```python
from build123d import *

# Parameters (mm, degrees)
SKETCH1_W           = 50
SKETCH1_H           = 39
BOSS_EXTRUDE1_DEPTH = 3
SKETCH2_W           = 2
SKETCH2_H           = 2
SKETCH2_H_2         = 8
SKETCH2_W_2         = 8
SKETCH2_W_3         = 10
SKETCH2_H_3         = 10
BOSS_EXTRUDE2_DEPTH = 5
SKETCH3_W           = 44
SKETCH3_H           = 28
CUT_EXTRUDE1_DEPTH  = 5
SKETCH4_W           = 2
SKETCH4_H           = 2
SKETCH4_H_2         = 5.5
SKETCH4_W_2         = 5.5
BOSS_EXTRUDE3_DEPTH = 5
SKETCH5_W           = 2
SKETCH5_H           = 5.5
SKETCH5_H_2         = 2
SKETCH5_W_2         = 5.5
BOSS_EXTRUDE4_DEPTH = 5
SKETCH6_W           = 38
SKETCH6_H           = 17
CUT_EXTRUDE2_DEPTH  = 5
SKETCH7_W           = 35
SKETCH7_H           = 24
CUT_EXTRUDE3_DEPTH  = 5


with BuildPart() as part:
    # Sketch1 → Boss-Extrude1 (new body)
    with BuildSketch(Plane.XY):
        Polygon((5, 47), (0, 47), (0, 0), (63, 0), (63, 47), (58, 47), align=None)
        Polygon((5, 79), (5, 47), (58, 47), (58, 79), (56.5, 79), (6.5, 79), align=None)
        with Locations((31.5, 98.5)):
            Rectangle(SKETCH1_W, SKETCH1_H)
    extrude(amount=BOSS_EXTRUDE1_DEPTH)

    # Sketch2 → Boss-Extrude2 (add)
    with BuildSketch(Plane.XY.offset(3)):
        Polygon((53, 45), (61, 45), (61, 47), (58, 47), (53, 47), align=None)
        with Locations((62, 46)):
            Rectangle(SKETCH2_W, SKETCH2_H)
        with Locations((62, 41)):
            Rectangle(SKETCH2_W, SKETCH2_H_2)
        with Locations((62, 6)):
            Rectangle(SKETCH2_W, SKETCH2_H_2)
        with Locations((62, 1)):
            Rectangle(SKETCH2_W, SKETCH2_H)
        with Locations((57, 1)):
            Rectangle(SKETCH2_W_2, SKETCH2_H)
        with Locations((5, 1)):
            Rectangle(SKETCH2_W_3, SKETCH2_H)
        with Locations((5, 46)):
            Rectangle(SKETCH2_W_3, SKETCH2_H)
        with Locations((1, 29)):
            Rectangle(SKETCH2_W, SKETCH2_H_3)
    extrude(amount=BOSS_EXTRUDE2_DEPTH)

    # Sketch3 → Cut-Extrude1 (cut)
    with BuildSketch(Plane.XY.offset(3)):
        with Locations((31.5, 23.5)):
            Rectangle(SKETCH3_W, SKETCH3_H)
    extrude(amount=-CUT_EXTRUDE1_DEPTH, mode=Mode.SUBTRACT)

    # Sketch4 → Boss-Extrude3 (add)
    with BuildSketch(Plane.XY.offset(3)):
        with Locations((6, 48)):
            Rectangle(SKETCH4_W, SKETCH4_H)
        with Locations((6, 51.75)):
            Rectangle(SKETCH4_W, SKETCH4_H_2)
        Polygon((7, 49), (7, 47), (10, 47), (12.5, 47), (12.5, 49), align=None)
        with Locations((6, 74.25)):
            Rectangle(SKETCH4_W, SKETCH4_H_2)
        Polygon((5, 79), (5, 77), (7, 77), (7, 79), (6.5, 79), align=None)
        with Locations((9.75, 78)):
            Rectangle(SKETCH4_W_2, SKETCH4_H)
        with Locations((53.25, 78)):
            Rectangle(SKETCH4_W_2, SKETCH4_H)
        Polygon((56, 77), (58, 77), (58, 79), (56.5, 79), (56, 79), align=None)
        with Locations((57, 74.25)):
            Rectangle(SKETCH4_W, SKETCH4_H_2)
        with Locations((57, 51.75)):
            Rectangle(SKETCH4_W, SKETCH4_H_2)
        with Locations((57, 48)):
            Rectangle(SKETCH4_W, SKETCH4_H)
        Polygon((53, 47), (56, 47), (56, 49), (50.5, 49), (50.5, 47), align=None)
    extrude(amount=BOSS_EXTRUDE3_DEPTH)

    # Sketch5 → Boss-Extrude4 (add)
    with BuildSketch(Plane.XY.offset(3)):
        with Locations((7.5, 83.75)):
            Rectangle(SKETCH5_W, SKETCH5_H)
        Polygon((8.5, 81), (8.5, 79), (12.5, 79), (14, 79), (14, 81), align=None)
        with Locations((7.5, 80)):
            Rectangle(SKETCH5_W, SKETCH5_H_2)
        Polygon((54.5, 79), (54.5, 81), (49, 81), (49, 79), (50.5, 79), align=None)
        with Locations((55.5, 80)):
            Rectangle(SKETCH5_W, SKETCH5_H_2)
        with Locations((55.5, 83.75)):
            Rectangle(SKETCH5_W, SKETCH5_H)
        with Locations((51.75, 117)):
            Rectangle(SKETCH5_W_2, SKETCH5_H_2)
        with Locations((55.5, 117)):
            Rectangle(SKETCH5_W, SKETCH5_H_2)
        with Locations((55.5, 113.25)):
            Rectangle(SKETCH5_W, SKETCH5_H)
        with Locations((11.25, 117)):
            Rectangle(SKETCH5_W_2, SKETCH5_H_2)
        with Locations((7.5, 117)):
            Rectangle(SKETCH5_W, SKETCH5_H_2)
        with Locations((7.5, 113.25)):
            Rectangle(SKETCH5_W, SKETCH5_H)
    extrude(amount=BOSS_EXTRUDE4_DEPTH)

    # Sketch6 → Cut-Extrude2 (cut)
    with BuildSketch(Plane.XY.offset(3)):
        with Locations((31.5, 63)):
            Rectangle(SKETCH6_W, SKETCH6_H)
    extrude(amount=-CUT_EXTRUDE2_DEPTH, mode=Mode.SUBTRACT)

    # Sketch7 → Cut-Extrude3 (cut)
    with BuildSketch(Plane.XY.offset(3)):
        with Locations((31.5, 98.5)):
            Rectangle(SKETCH7_W, SKETCH7_H)
    extrude(amount=-CUT_EXTRUDE3_DEPTH, mode=Mode.SUBTRACT)


solid = part.part
```
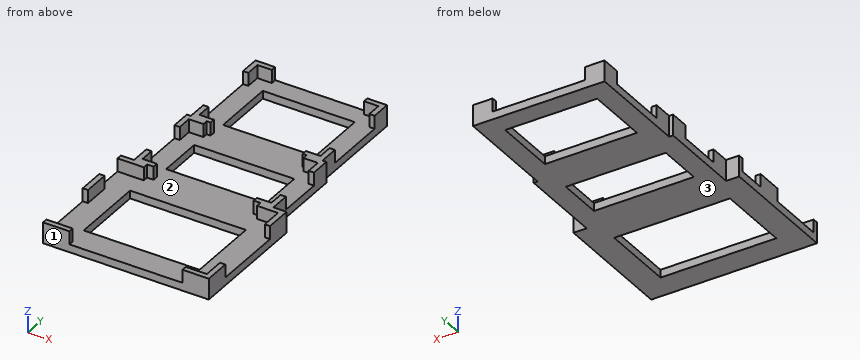
Work out the finished part from the listing and answer in its coordinate system (mm). Face numbers are marked on the shaded views. Round coordinates to 2 decimals unless told otherwise and drop trailing zeros. Loops run counter-clockwise (first coordinate to the right, second up) from the corner with the lowest first, then second, coordinate; pieces in that order, holes last.
(1) Each of these flat-tipped pins is pushed along its axis until it touches: P1, Ø2.5, axis at y = 99.5, z = 4, coming from the -X side; P2, Ø2.5, axis at y = 75.5, z = 4.5, coming from the +X side; P3, Ø2, axis at y = 41.5, z = 6, coming from the -X side. Where does it stop, or does it pass through?
Computed values:
P1: stops at x = 6.5
P2: stops at x = 58
P3: stops at x = 61
(2) The part is cut by section D-D, the plane y = 97. Give the vertices of the cut face in (x, z), and give its area (3 significant figures).
Computed values:
outline: (6.5, 0) - (14, 0) - (14, 3) - (6.5, 3) - close; (49, 0) - (56.5, 0) - (56.5, 3) - (49, 3) - close
area: 45.0 mm2
(3) The part is cut by section A-A, the plane y = 18.5. Give the vertices of the cut face in (x, z), and give its area (3 significant figures).
Computed values:
outline: (0, 0) - (9.5, 0) - (9.5, 3) - (0, 3) - close; (53.5, 0) - (63, 0) - (63, 3) - (53.5, 3) - close
area: 57.0 mm2
(4) The part is cut by section C-C, the plane z = 6.75. Give the number of separate pieces and of enclosed holes in the cut face, and give its area (3 significant figures).
Computed values:
separate pieces: 9
enclosed holes: 0
area: 340 mm2
(5) The mould has two halves that part along Y. Classify the marked faces 1, 2 and 3: pulls with the +Y half, pulls with the -Y half, needs draft (parallel to the pull), parting line crosses it, or undercut.
Computed values:
face 1: pulls with the -Y half
face 2: undercut
face 3: needs draft
(6) The part is cut by section B-B, the plane x = 26. Give the vertices of the cut face in (y, z).
Computed values:
outline: (0, 0) - (9.5, 0) - (9.5, 3) - (0, 3) - close; (37.5, 0) - (54.5, 0) - (54.5, 3) - (37.5, 3) - close; (71.5, 0) - (86.5, 0) - (86.5, 3) - (71.5, 3) - close; (110.5, 0) - (118, 0) - (118, 3) - (110.5, 3) - close
(7) Find the intervals of material crossed by L1, parallel to Y at x = 7.5, z = 5.75; L2, parallel to Y at x = 21, z = 2.5; L3, parallel to Y at x = 52, z = 6, in increasing order.
Computed values:
L1: y = 0 to 2, 45 to 49, 77 to 86.5, 110.5 to 118
L2: y = 0 to 9.5, 37.5 to 54.5, 71.5 to 86.5, 110.5 to 118
L3: y = 47 to 49, 77 to 81, 116 to 118
